The model under review builds one solid part; all positions refer to its coordinate system, in mm. A direction names the side the tool comes from. Round coordinates to 2 decimals unless told otherwise and drop trailing zeros. Loops run counter-clockwise (first coordinate to the right, second up) from the corner with the lowest first, then second, coordinate; pieces in that order, holes last. Notation, with made-up numbers: M 86,42 L 124,42 A18 ccw 124,77 Z; hole C 82.25,-22 d3. An arc over 180 degrees is marked long. Use a Markdown table: item, result. Add a question column.
```python
from build123d import *
from build123d.topology import SkipClean

# Parameters (mm, degrees)
SALIENTE_EXTRUIR1_DEPTH = 17
CROQUIS4_R              = 2.5
CORTAR_EXTRUIR2_DEPTH   = 5
CROQUIS5_W              = 27
CROQUIS5_H              = 17
CROQUIS5_R              = 2.5
SALIENTE_EXTRUIR4_DEPTH = 7
REDONDEO2_R             = 2
CROQUIS6_R              = 3.5
CORTAR_EXTRUIR3_DEPTH   = 1
CROQUIS9_R              = 3.5
SALIENTE_EXTRUIR7_DEPTH = 10
CROQUIS10_W             = 20
CROQUIS10_H             = 25
SALIENTE_EXTRUIR8_DEPTH = 10
CROQUIS11_R             = 2.3
CORTAR_EXTRUIR6_DEPTH   = 10
CROQUIS12_R             = 3.5
CORTAR_EXTRUIR7_DEPTH   = 4
REDONDEO3_R             = 2
CROQUIS8_R              = 1.1
CORTAR_EXTRUIR8_DEPTH   = 41.770700264


with BuildPart() as part:
    # Croquis2 → Saliente-Extruir1 (new body)
    with BuildSketch(Plane.XY):
        Polygon((0, 0), (0, 11.5), (5, 11.5), (5, 0), (28, 0), (28, 11.5), (33, 11.5), (33, 0), (33, -3), (0, -3), align=None)
    extrude(amount=SALIENTE_EXTRUIR1_DEPTH)

    # Croquis4 → Cortar-Extruir2 (cut)
    with BuildSketch(Plane(origin=(0, 0, 0), x_dir=(1, 0, 0), z_dir=(0, 1, 0))):
        with Locations(Location((9, -8.5, 0), (0, 0, 270))):
            Circle(CROQUIS4_R)
        with Locations(Location((24, -8.5, 0), (0, 0, 270))):
            Circle(CROQUIS4_R)
    extrude(amount=-CORTAR_EXTRUIR2_DEPTH, mode=Mode.SUBTRACT)

    # Croquis5 → Saliente-Extruir4 (add)
    with SkipClean():  # the faces are left unmerged after this step: merging them gives an invalid solid
        with BuildSketch(Plane.XZ.offset(3)):
            with Locations((16.5, 8.5)):
                Rectangle(CROQUIS5_W, CROQUIS5_H)
            with Locations(Location((9, 8.5, 0), (0, 0, 90))):
                Circle(CROQUIS5_R, mode=Mode.SUBTRACT)
            with Locations(Location((24, 8.5, 0), (0, 0, 270))):
                Circle(CROQUIS5_R, mode=Mode.SUBTRACT)
        extrude(amount=SALIENTE_EXTRUIR4_DEPTH)
    add(part.part.scale(1), mode=Mode.REPLACE)  # the faces are merged on a copy

    # Redondeo2
    redondeo2_edges = [part.edges().sort_by_distance(p)[0] for p in [
        (30, -3, 8.5),
        (3, -3, 8.5),
    ]]
    fillet(redondeo2_edges, radius=REDONDEO2_R)

    # Croquis6 → Cortar-Extruir3 (cut)
    with SkipClean():  # the faces are left unmerged after this step: merging them gives an invalid solid
        with BuildSketch(Plane(origin=(0, 0, 0), x_dir=(1, 0, 0), z_dir=(0, 1, 0))):
            with Locations(Location((9, -8.5, 0), (0, 0, 270))):
                Circle(CROQUIS6_R)
            with Locations(Location((24, -8.5, 0), (0, 0, 270))):
                Circle(CROQUIS6_R)
        extrude(amount=-CORTAR_EXTRUIR3_DEPTH, mode=Mode.SUBTRACT)

    # Croquis9 → Saliente-Extruir7 (add)
    with BuildSketch(Plane(origin=(0, 0, 0), x_dir=(1, 0, 0), z_dir=(0, 1, 0))):
        with Locations((9, -8.5)):
            Circle(CROQUIS9_R)
        with Locations((24, -8.5)):
            Circle(CROQUIS9_R)
    extrude(amount=-SALIENTE_EXTRUIR7_DEPTH)

    # Croquis10 → Saliente-Extruir8 (add)
    with BuildSketch(Plane.XZ.offset(10)):
        with Locations((16.5, 8.5)):
            Rectangle(CROQUIS10_W, CROQUIS10_H)
    extrude(amount=-SALIENTE_EXTRUIR8_DEPTH)

    # Croquis11 → Cortar-Extruir6 (cut)
    with BuildSketch(Plane.XZ.offset(10)):
        with Locations(Location((16.5, 14.5, 0), (0, 0, 270))):
            Circle(CROQUIS11_R)
        with Locations(Location((16.5, 2.5, 0), (0, 0, 270))):
            Circle(CROQUIS11_R)
    extrude(amount=-CORTAR_EXTRUIR6_DEPTH, mode=Mode.SUBTRACT)

    # Croquis12 → Cortar-Extruir7 (cut)
    with BuildSketch(Plane(origin=(0, 0, 0), x_dir=(1, 0, 0), z_dir=(0, 1, 0))):
        with Locations(Location((16.5, -2.5, 0), (0, 0, 270))):
            Circle(CROQUIS12_R)
        with Locations(Location((16.5, -14.5, 0), (0, 0, 270))):
            Circle(CROQUIS12_R)
    extrude(amount=-CORTAR_EXTRUIR7_DEPTH, mode=Mode.SUBTRACT)

    # Redondeo3
    redondeo3_edges = [part.edges().sort_by_distance(p)[0] for p in [
        (6.5, -5, -4),
        (6.5, -5, 21),
        (26.5, -5, 21),
        (26.5, -5, -4),
    ]]
    fillet(redondeo3_edges, radius=REDONDEO3_R)

    # Croquis8 → Cortar-Extruir8 (cut, through all)
    with BuildSketch(Plane.XY.offset(17)):
        with Locations((2.5, 5.75)):
            Circle(CROQUIS8_R)
        with Locations((30.5, 5.75)):
            Circle(CROQUIS8_R)
    extrude(amount=-CORTAR_EXTRUIR8_DEPTH, mode=Mode.SUBTRACT)


solid = part.part
```
(1) Draft analysis for pull direction Y (two halves, no side actions). For faces 1 (the face through (3.55, 6.08, 8.62)), 2 (the face through (16, -4, 17)), 3 (the face through (14.255, -7.042, 2.999)), state which applies: released by +Y, released by -Y, zero draft, split by the parting line, or undercut.
(2) Consider section C-C, the plane z = 14.5. Give the boundary of the cut face in (x, y), then the cut area to 3 significant figures.
(3) Consider section A-A, the plane y = 5.75. Give the boundary of the cut face in (x, z).
(4) For faces 4 (the face through (30, 1, 17)), 5 (the face through (19.45, -1.97, 16.38)), 6 (the face through (3, 1, 0)), 7 (the face through (26.5, -5, -1)), list the 3-axis set-ups (+Z, -Z, +X, -X, +Y, -Y) from which the entire face can be reached by the end or side of a thin tool; tool diameter is ignored.
(5) Consider section B-B, the plane x = 16.5. Give the boundary of the cut face in (y, z).
(6) Insertion check: pin 1 Ø8 at (x, z) = (16.5, 2.5) entering from +Y; pin 2 Ø1.6 at (y, z) = (-5.5, 17.5) entering from -X; pin 3 Ø12 at (x, y) = (8, 8.5) entering from -Z. Each pin has a flat end and moves straight along its axis. Give the tip position at first contact, or say it passes through.
(7) Consider section D-D, the plane y = -7. Give the boundary of the cut face in (x, z), then the cut area to 3 significant figures.
(8) To check wall thickness, follow probe 1 along X at (y, z) = (10.75, 2.5); probe 2 along Z at (x, y) = (15, -9); probe 3 along X at (y, z) = (-1.3, 14.5). State the ranges of each line that lie inside material, in increasing order.
Found:
| question | item | result |
|---|---|---|
| 1 | face 1 | undercut |
| 1 | face 2 | released by +Y |
| 1 | face 3 | zero draft |
| 2 | outline | M 0,-3 L 1,-3 A2 cw 3,-5 L 3,-10 L 14.2,-10 L 14.2,-4 L 13,-4 L 13,0 L 5,0 L 5,11.5 L 0,11.5 Z; M 18.8,-10 L 30,-10 L 30,-5 A2 cw 32,-3 L 33,-3 L 33,11.5 L 28,11.5 L 28,0 L 20,0 L 20,-4 L 18.8,-4 Z; hole C 2.5,5.75 d2.2; hole C 30.5,5.75 d2.2 |
| 2 | area | 342 mm^2 |
| 3 | outline | M 0,0 L 1.4,0 L 1.4,17 L 0,17 Z; M 3.6,0 L 5,0 L 5,17 L 3.6,17 Z; M 28,0 L 29.4,0 L 29.4,17 L 28,17 Z; M 31.6,0 L 33,0 L 33,17 L 31.6,17 Z |
| 4 | face 4 | +Z, +X, +Y, -Y |
| 4 | face 5 | +Y |
| 4 | face 6 | -Z, -X, +Y, -Y |
| 4 | face 7 | -Z, +X, +Y, -Y |
| 5 | outline | M -10,-4 L 0,-4 L 0,-1 L -4,-1 L -4,0.2 L -10,0.2 Z; M -10,4.8 L -4,4.8 L -4,6 L 0,6 L 0,11 L -4,11 L -4,12.2 L -10,12.2 Z; M -10,16.8 L -4,16.8 L -4,18 L 0,18 L 0,21 L -10,21 Z |
| 6 | pin 1 | stops at y = 0 |
| 6 | pin 2 | stops at x = 3 |
| 6 | pin 3 | stops at z = 0 |
| 7 | outline | M 3,0 L 6.5,0 L 6.5,-2 A2 ccw 8.5,-4 L 24.5,-4 A2 ccw 26.5,-2 L 26.5,0 L 30,0 L 30,17 L 26.5,17 L 26.5,19 A2 ccw 24.5,21 L 8.5,21 A2 ccw 6.5,19 L 6.5,17 L 3,17 Z; hole C 16.5,2.5 d4.6; hole C 16.5,14.5 d4.6 |
| 7 | area | 582 mm^2 |
| 8 | probe 1 | x = 0 to 5, 28 to 33 |
| 8 | probe 2 | z = -4 to 0.76, 4.24 to 12.76, 16.24 to 21 |
| 8 | probe 3 | x = 0 to 13, 20 to 33 |
